Model file for the job. Use its own axes, mm. A direction names the side the tool comes from. Coordinates: 2 decimals unless noted, no trailing zeros. Write each loop counter-clockwise with the first axis right and the second up, starting at its lowest first coordinate (ties: lowest second). Pieces come first, ordered by that corner, then holes. Notation, with made-up numbers: M 56,69 L 106,69 A11 cw 106,80 Z; hole C 42.5,60 d11. An arc over 180 degrees is marked long. Put each result on its own line as item: value. Start each with the question number.
Q1. Drill centre lines: line 1 along Z through (x, y) = (36, 15.4); line 2 along Z through (x, y) = (19.5, 15.6); line 3 along Z through (x, y) = (36, -17). Where is each one in solid material? Low to high.
Q2. Cut at A-A (x = -20). Write the cut outline in (y, z), then the cut area to 3 significant figures.
Q3. Pull direction Y, two halves, no side cores. Call faces 6 (the cylindrical face through (28.649, -16.486, 24.323)), 7 (the flat face through (36, -15.5, 5)), 8 (the cylindrical face through (-2.285, 3.584, 20.874)), 9 (the flat face through (36, 15.5, 5)): pulls with the +Y half, pulls with the -Y half, needs draft (parallel to the pull), parting line crosses it, or undercut.
Q4. Cut at B-B (y = 0). Write the cut outline in (x, z), then the cut area to 3 significant figures.
Q5. Drop flat-ended pins along their axis: pin 1 (4.5 mm diameter, centred on x = 36, z = 3, fed in from -Y); pin 2 (5 mm diameter, centred on x = 36, z = 3, fed in from +Y); pin 3 (10.5 mm diameter, centred on x = -12, y = -2, fed in from -Z); pin 4 (1.9 mm diameter, centred on x = 14, z = 35.5, fed in from -Y). Give the stop position or say it passes through.
Q6. Cut at C-C (z = 20). Write the cut outline in (x, y), then the cut area to 3 significant figures.
Q7. Cut at D-D (z = 3). Give the number of separate pieces and of enclosed holes in the cut face, then the cut area to 3 significant figures.
Q8. Which spindle directions (+Z, -Z, +X, -X, +Y, -Y) get a long thin tool onto all of the face, cutting with end or side? Do faces 1 (the flat face through (3, -4, 12)), 2 (the flat face through (10, -14, -5)), 3 (the flat face through (25, 9, 15)), 4 (the cylindrical face through (26.3, 16.5, 2.9)), 5 (the flat face through (25.2, 11.5, 14.6)). Say none if no direction does.
```python
from build123d import *

# Parameters (mm, degrees)
SKETCH_1_W               = 50
SKETCH_1_H               = 35
EXTRUDE_1_DEPTH          = 30
HOLE_WIZARD_394_D        = 8.5
HOLE_WIZARD_498_D        = 3.2
HOLE_WIZARD_652_D        = 15
CHAMFER_1_SIZE           = 1
CHAMFER_1_SIZE_2         = 0.708203932
SKETCH_9_W               = 30
SKETCH_9_H               = 6
EXTRUDE_3_DEPTH          = 15
SKETCH_10_W              = 6
SKETCH_10_H              = 23
EXTRUDE_4_DEPTH          = 9
HOLE_WIZARD_1_D          = 3.2
HOLE_WIZARD_1_DEPTH      = 6
MIRROR_2_COPY_1_D        = 3.2
MIRROR_2_COPY_1_DEPTH    = 6
SKETCH_15_W              = 30
SKETCH_15_H              = 6
EXTRUDE_6_DEPTH          = 10
HOLE_WIZARD_2_D          = 3.2
MIRROR_5_COPY_1_D        = 3.2
MIRROR_6_COPY_1_D        = 3.2
MIRROR_6_COPY_2_SKETCH_W = 30
MIRROR_6_COPY_2_SKETCH_H = 6
MIRROR_6_COPY_2_DEPTH    = 10
MIRROR_6_COPY_3_D        = 3.2
MIRROR_6_COPY_4_D        = 3.2
HOLE_WIZARD_3_D          = 5.4
HOLE_WIZARD_3_DEPTH      = 2
HOLE_WIZARD_4_D          = 12
HOLE_WIZARD_4_DEPTH      = 12


with BuildPart() as part:
    # 草图1 → 凸台-拉伸1 (new body)
    with BuildSketch(Plane.XY):
        Rectangle(SKETCH_1_W, SKETCH_1_H)
    extrude(amount=EXTRUDE_1_DEPTH)

    # Hole Wizard 394 (through all)
    with Locations(Plane.XY.offset(30)):
        with Locations((0, 0)):
            Hole(HOLE_WIZARD_394_D / 2)

    # Hole Wizard 498 (through all)
    with Locations(Plane.XY.offset(30)):
        with Locations((8, 0), (0, 8), (-8, 0), (0, -8)):
            Hole(HOLE_WIZARD_498_D / 2)

    # Hole Wizard 652 (through all)
    with Locations(Plane.XY.offset(30)):
        with Locations((20, 0), (-20, 0)):
            Hole(HOLE_WIZARD_652_D / 2)

    # 倒角1
    # the kernel refuses this chamfer: 1, 0.708203932 mm, written as the material it takes off along each edge
    with BuildSketch(Plane(origin=(-20, 0, 0), x_dir=(-0.8790200859122482, 0.4767847402789059, 0), z_dir=(-0.4767847402789059, -0.8790200859122482, 0))) as chamfer_1_piece_1:
        Polygon((7.5, -CHAMFER_1_SIZE), (7.5 + CHAMFER_1_SIZE, 0), (7.5, 0), align=None)
    revolve(axis=Axis((-20, 0, 0), (0, 0, -1)), revolution_arc=303.048763938, mode=Mode.SUBTRACT)
    with BuildSketch(Plane(origin=(-20, 0, 30), x_dir=(-0.879020085912248, 0.47678474027890627, 0), z_dir=(-0.47678474027890627, -0.879020085912248, 0))) as chamfer_1_piece_2:
        Polygon((7.5 + CHAMFER_1_SIZE, 0), (7.5, CHAMFER_1_SIZE), (7.5, 0), align=None)
    revolve(axis=Axis((-20, 0, 30), (0, 0, -1)), revolution_arc=303.048763938, mode=Mode.SUBTRACT)
    with BuildSketch(Plane(origin=(20, 0, 30), x_dir=(0.879020085912248, -0.4767847402789061, 0), z_dir=(0.4767847402789061, 0.879020085912248, 0))) as chamfer_1_piece_3:
        Polygon((7.5 + CHAMFER_1_SIZE, 0), (7.5, CHAMFER_1_SIZE), (7.5, 0), align=None)
    revolve(axis=Axis((20, 0, 30), (0, 0, -1)), revolution_arc=303.048763938, mode=Mode.SUBTRACT)
    with BuildSketch(Plane(origin=(20, 0, 0), x_dir=(0.8790200859122481, 0.476784740278906, 0), z_dir=(0.476784740278906, -0.8790200859122481, 0))) as chamfer_1_piece_4:
        Polygon((7.5, CHAMFER_1_SIZE), (7.5 + CHAMFER_1_SIZE, 0), (7.5, 0), align=None)
    revolve(axis=Axis((20, 0, 0), (0, 0, 1)), revolution_arc=303.048763938, mode=Mode.SUBTRACT)
    with BuildSketch(Plane(origin=(-25, 5.590169944, 32.778051389), x_dir=(0.7914486393779661, 0.611235675682274, 0), z_dir=(0, 0, -1)), Plane(origin=(25, -5.590169944, 32.778051389), x_dir=(-0.7914486393779661, -0.611235675682274, 0), z_dir=(0, 0, -1))) as chamfer_1_piece_5:
        with BuildLine():
            Line((1.080663788, 0), (CHAMFER_1_SIZE_2 * 0.611235676113, -CHAMFER_1_SIZE_2 * 0.791448639936))
            Line((CHAMFER_1_SIZE_2 * 0.611235676113, -CHAMFER_1_SIZE_2 * 0.791448639936), (0, 0))
            ThreePointArc((0, 0), (0.555522087, -0.019473843), (1.080663788, 0))
        make_face()
    extrude(amount=35.556102778, mode=Mode.SUBTRACT)
    with BuildSketch(Plane(origin=(-25, -5.590169944, 32.778051389), x_dir=(0.7914486393779665, -0.6112356756822735, 0), z_dir=(0, 0, -1))) as chamfer_1_piece_6:
        with BuildLine():
            Line((1.080663788, 0), (CHAMFER_1_SIZE_2 * 0.611235676113, CHAMFER_1_SIZE_2 * 0.791448639936))
            Line((CHAMFER_1_SIZE_2 * 0.611235676113, CHAMFER_1_SIZE_2 * 0.791448639936), (0, 0))
            ThreePointArc((0, 0), (0.555522087, 0.019473843), (1.080663788, 0))
        make_face()
    extrude(amount=35.556102778, mode=Mode.SUBTRACT)
    with BuildSketch(Plane(origin=(25, 5.590169944, 32.778051389), x_dir=(0, 1, 0), z_dir=(0, 0, -1))) as chamfer_1_piece_7:
        with BuildLine():
            Line((CHAMFER_1_SIZE_2, 0), (0.660540261, -0.855289885))
            ThreePointArc((0.660540261, -0.855289885), (0.354967464, -0.427764092), (0, 0))
            Line((0, 0), (CHAMFER_1_SIZE_2, 0))
        make_face()
    extrude(amount=35.556102778, mode=Mode.SUBTRACT)

    # 草图9 → 凸台-拉伸3 (add)
    with BuildSketch(Plane(origin=(25, 0, 0), x_dir=(0, 0, -1), z_dir=(1, 0, 0))):
        with Locations((-15, 14.5)):
            Rectangle(SKETCH_9_W, SKETCH_9_H)
        with Locations((-15, -14.5)):
            Rectangle(SKETCH_9_W, SKETCH_9_H)
    extrude(amount=EXTRUDE_3_DEPTH)

    # 草图10 → 凸台-拉伸4 (add, symmetric)
    with BuildSketch(Plane.XY.offset(15)):
        with Locations((37, 0)):
            Rectangle(SKETCH_10_W, SKETCH_10_H)
    extrude(amount=EXTRUDE_4_DEPTH, both=True)

    # 孔1
    with Locations(Plane(origin=(0, 11.5, 0), x_dir=(-1, 0, 0), z_dir=(0, -1, 0))):
        with Locations((-36, -3), (-29, -3)):
            hole_wizard_1 = Hole(HOLE_WIZARD_1_D / 2, depth=HOLE_WIZARD_1_DEPTH)

    # 镜向1: 孔1 across plane
    add(hole_wizard_1.mirror(Plane.XY.offset(15)), mode=Mode.SUBTRACT)

    # 镜向2: 孔1 across plane
    add(hole_wizard_1.mirror(Plane(origin=(0, 0, 0), x_dir=(0, 0, 1), z_dir=(0, -1, 0))), mode=Mode.SUBTRACT)

    # 镜向2 copy 1
    with Locations(Plane(origin=(0, -11.5, 30), x_dir=(-1, 0, 0), z_dir=(0, 1, 0))):
        with Locations((-36, -3), (-29, -3)):
            Hole(MIRROR_2_COPY_1_D / 2, depth=MIRROR_2_COPY_1_DEPTH)

    # 草图15 → 凸台-拉伸6 (add)
    with BuildSketch(Plane(origin=(0, 0, 0), x_dir=(-1, 0, 0), z_dir=(0, 0, -1))):
        with Locations((-25, 14.5)):
            Rectangle(SKETCH_15_W, SKETCH_15_H)
    extrude_6 = extrude(amount=EXTRUDE_6_DEPTH)

    # 孔2 (through all)
    with Locations(Plane(origin=(0, 11.5, 0), x_dir=(-1, 0, 0), z_dir=(0, -1, 0))):
        with Locations((-19.5, 5.5), (-14, 5.5), (-25, 5.5)):
            hole_wizard_2 = Hole(HOLE_WIZARD_2_D / 2)

    # 镜向4: 孔2 across plane
    add(hole_wizard_2.mirror(Plane(origin=(25, 0, 0), x_dir=(0, 0, 1), z_dir=(1, 0, 0))), mode=Mode.SUBTRACT)

    # 镜向5: 凸台-拉伸6, 孔2 across plane
    add(extrude_6.mirror(Plane.XY.offset(15)))
    add(hole_wizard_2.mirror(Plane.XY.offset(15)), mode=Mode.SUBTRACT)

    # 镜向5 copy 1 (through all)
    with Locations(Plane(origin=(50, 11.5, 30), x_dir=(1, 0, 0), z_dir=(0, -1, 0))):
        with Locations((-19.5, 5.5), (-14, 5.5), (-25, 5.5)):
            Hole(MIRROR_5_COPY_1_D / 2)

    # 镜向6: 凸台-拉伸6, 孔2 across plane
    add(extrude_6.mirror(Plane(origin=(0, 0, 0), x_dir=(0, 0, 1), z_dir=(0, -1, 0))))
    add(hole_wizard_2.mirror(Plane(origin=(0, 0, 0), x_dir=(0, 0, 1), z_dir=(0, -1, 0))), mode=Mode.SUBTRACT)

    # 镜向6 copy 1 (through all)
    with Locations(Plane(origin=(50, -11.5, 0), x_dir=(1, 0, 0), z_dir=(0, 1, 0))):
        with Locations((-19.5, 5.5), (-14, 5.5), (-25, 5.5)):
            Hole(MIRROR_6_COPY_1_D / 2)

    # 镜向6 copy 2 sketch → 镜向6 copy 2 (add)
    with BuildSketch(Plane(origin=(0, 0, 30), x_dir=(-1, 0, 0), z_dir=(0, 0, 1))):
        with Locations((-25, 14.5)):
            Rectangle(MIRROR_6_COPY_2_SKETCH_W, MIRROR_6_COPY_2_SKETCH_H)
    extrude(amount=MIRROR_6_COPY_2_DEPTH)

    # 镜向6 copy 3 (through all)
    with Locations(Plane(origin=(0, -11.5, 30), x_dir=(-1, 0, 0), z_dir=(0, 1, 0))):
        with Locations((-19.5, 5.5), (-14, 5.5), (-25, 5.5)):
            Hole(MIRROR_6_COPY_3_D / 2)

    # 镜向6 copy 4 (through all)
    with Locations(Plane(origin=(50, -11.5, 30), x_dir=(1, 0, 0), z_dir=(0, 1, 0))):
        with Locations((-19.5, -5.5), (-14, -5.5), (-25, -5.5)):
            Hole(MIRROR_6_COPY_4_D / 2)

    # 孔3
    with Locations(Plane(origin=(0, -17.5, 0), x_dir=(-1, 0, 0), z_dir=(0, -1, 0))):
        with Locations((-29, -3), (-36, -3), (-36, -27), (-29, -27)):
            hole_wizard_3 = Hole(HOLE_WIZARD_3_D / 2, depth=HOLE_WIZARD_3_DEPTH)

    # 镜向7: 孔3 across plane
    add(hole_wizard_3.mirror(Plane(origin=(0, 0, 0), x_dir=(0, 0, 1), z_dir=(0, -1, 0))), mode=Mode.SUBTRACT)

    # 孔4
    with Locations(Plane(origin=(0, 0, 0), x_dir=(-1, 0, 0), z_dir=(0, 0, -1))):
        with Locations((0, 0)):
            Hole(HOLE_WIZARD_4_D / 2, depth=HOLE_WIZARD_4_DEPTH)


solid = part.part
```
Computed values:
1. line 1: -10 to -7.1, -3.9 to 1.4, 4.6 to 25.4, 28.6 to 33.9, 37.1 to 40
1. line 2: -10 to -7.1, -3.9 to 33.9, 37.1 to 40
1. line 3: -10 to -7.1, -3.9 to 0.3, 5.7 to 24.3, 29.7 to 33.9, 37.1 to 40
2. outline: M -17.5,0 L -8.5,0 L -7.5,1 L -7.5,29 L -8.5,30 L -17.5,30 Z; M 7.5,1 L 8.5,0 L 17.5,0 L 17.5,30 L 8.5,30 L 7.5,29 Z
2. area: 598 mm2
3. face 6: needs draft
3. face 7: pulls with the -Y half
3. face 8: undercut
3. face 9: pulls with the +Y half
4. outline: M -12.5,1 L -11.5,0 L -9.6,0 L -9.6,30 L -11.5,30 L -12.5,29 Z; M -6.4,0 L -6,0 L -6,12 L -4.25,12 L -4.25,30 L -6.4,30 Z; M 4.25,12 L 6,12 L 6,0 L 6.4,0 L 6.4,30 L 4.25,30 Z; M 9.6,0 L 11.5,0 L 12.5,1 L 12.5,29 L 11.5,30 L 9.6,30 Z; M 34,6 L 40,6 L 40,24 L 34,24 Z
4. area: 367 mm2
5. pin 1: y = -15.5
5. pin 2: y = 15.5
5. pin 3: z = 0
5. pin 4: through
6. outline: M -25,-17.5 L 40,-17.5 L 40,17.5 L -25,17.5 L -25,6.3 L -24.14,6.25 A7.5 cw long -24.14,-6.25 L -25,-6.3 Z; hole C -8,0 d3.2; hole C 0,0 d8.5; hole C 0,-8 d3.2; hole C 0,8 d3.2; hole C 8,0 d3.2; hole M 24.14,-6.25 L 25,-6.3 L 25,-11.5 L 34,-11.5 L 34,11.5 L 25,11.5 L 25,6.3 L 24.14,6.25 A7.5 ccw long Z
6. area: 1,660 mm2
7. separate pieces: 5
7. enclosed holes: 5
7. area: 1,370 mm2
8. face 1: -Z
8. face 2: -Z, -X, +Y, -Y
8. face 3: +Z, -Z
8. face 4: +Y
8. face 5: none
